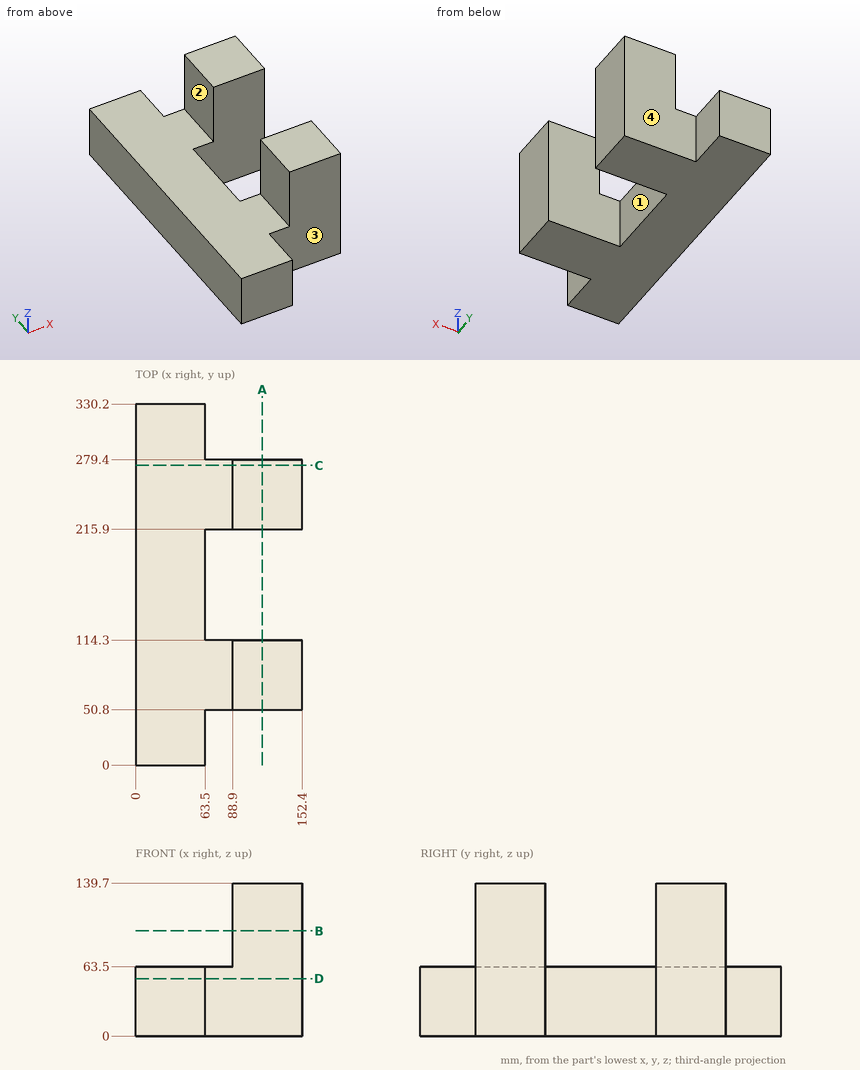
Answer from the drawing. Dimensions are ordinates in mm from the lowest x, y and z of the part. A direction names the side the tool comes from. Give positions to 0.01 mm unless a question says otherwise; leave off trailing zeros. Order: outer loops, then holes, each group sorted by start corner. A loop starts at its lowest first (then second) coordinate and runs counter-clockwise, first axis right, second up.
(1) Straight lines are drawn through the part: L1, parallel to Y at x = 97, z = 90.5; L2, parallel to Z at x = 23, y = 226.5. For each, find the intervals that lie inside material, in ascending order.
(2) Given pin 1 (2 mm diameter, centred on x = 93.5, z = 37, fed in from -Y); pin 2 (19 mm diameter, centred on y = 67.5, z = 102, fed in from -X), each flat-ended and moving along its own axis, determine where each tip first touches the part or whether it passes through.
(3) Find section D-D (z = 52.5). Give the vertices of the cut face in (x, y).
(4) Find section C-C (y = 274). Give the vertices of the cut face in (x, z), plus the area to 3 significant figures.
(5) Find section A-A (x = 116). Give the vertices of the cut face in (y, z), plus the area to 3 significant figures.
(6) Find section B-B (z = 96). Give the vertices of the cut face in (x, y), plus the area to 3 significant figures.
(7) For the marked faces 1, 2, 3 and 4, determine the directions among +Z, -Z, +X, -X, +Y, -Y from which every point of the face is accessible in a straight line to the end or side of a thin tool.
Result sheet:
1. L1: y = 50.8 to 114.3, 215.9 to 279.4
1. L2: z = 0 to 63.5
2. pin 1: stops at y = 50.8
2. pin 2: stops at x = 88.9
3. outline: (0, 0) - (63.5, 0) - (63.5, 50.8) - (152.4, 50.8) - (152.4, 114.3) - (63.5, 114.3) - (63.5, 215.9) - (152.4, 215.9) - (152.4, 279.4) - (63.5, 279.4) - (63.5, 330.2) - (0, 330.2) - close
4. outline: (0, 0) - (152.4, 0) - (152.4, 139.7) - (88.9, 139.7) - (88.9, 63.5) - (0, 63.5) - close
4. area: 14,500 mm2
5. outline: (50.8, 0) - (114.3, 0) - (114.3, 139.7) - (50.8, 139.7) - close; (215.9, 0) - (279.4, 0) - (279.4, 139.7) - (215.9, 139.7) - close
5. area: 17,700 mm2
6. outline: (88.9, 50.8) - (152.4, 50.8) - (152.4, 114.3) - (88.9, 114.3) - close; (88.9, 215.9) - (152.4, 215.9) - (152.4, 279.4) - (88.9, 279.4) - close
6. area: 8,060 mm2
7. face 1: +Z, -Z, +X
7. face 2: +Z, -X, +Y, -Y
7. face 3: +Z, -Z, +X, -Y
7. face 4: +Z, -Z, +X, +Y
